Can you work these out from the model? Positions are in its coordinate system, mm. A direction names the side the tool comes from. Round coordinates to 2 decimals unless told otherwise and drop trailing zeros. Order: outer loops, then holes, each group sorted by start corner. A loop starts at its lowest first (then second) coordinate and runs counter-clockwise, first axis right, second up. Notation, with made-up numbers: (19, -8.75) - (34, -8.75) arc R21 ccw to (34, 5.25) - close; hole circle Ø6 at (-18.5, 32.25). An arc over 180 degrees is marked (long way). Write item = value, one per line.
from build123d import *

# Parameters (mm, degrees)
EXTRUDE_1_DEPTH        = 40
SKETCH_5_W             = 3
SKETCH_5_H             = 6
SKETCH_5_W_2           = 6
SKETCH_5_H_2           = 3
EXTRUDE_3_DEPTH        = 2.5
SKETCH_6_W             = 6
SKETCH_6_H             = 3
SKETCH_6_W_2           = 3
SKETCH_6_H_2           = 6
EXTRUDE_4_DEPTH        = 2.5
FILLET_1_R             = 1
CUT_EXTRUDE_8754_DEPTH = 7
CUT_EXTRUDE_START      = -7
CUT_EXTRUDE_9199_DEPTH = 7


with BuildPart() as part:
    # 草图2 → 凸台-拉伸1 (new body)
    with BuildSketch(Plane(origin=(0, 0, 0), x_dir=(1, 0, 0), z_dir=(0, 1, 0))):
        with BuildLine():
            Line((-33, 3.25), (-36.5, 3.25))
            Line((-36.5, 3.25), (-36.5, -3.25))
            Line((-36.5, -3.25), (-33, -3.25))
            ThreePointArc((-33, -3.25), (-34.3699608, -13.457697281), (-37.384420147, -23.305890579))
            ThreePointArc((-37.384420147, -23.305890579), (-35.741677738, -34.13030337), (-25.5, -38))
            Line((-25.5, -38), (-25.5, -41.5))
            Line((-25.5, -41.5), (-19, -41.5))
            Line((-19, -41.5), (-19, -38))
            ThreePointArc((-19, -38), (0, -34.737686486), (19, -38))
            Line((19, -38), (19, -41.5))
            Line((19, -41.5), (25.5, -41.5))
            Line((25.5, -41.5), (25.5, -38))
            ThreePointArc((25.5, -38), (35.741677738, -34.13030337), (37.384420147, -23.305890579))
            ThreePointArc((37.384420147, -23.305890579), (34.3699608, -13.457697281), (33, -3.25))
            Line((33, -3.25), (36.5, -3.25))
            Line((36.5, -3.25), (36.5, 3.25))
            Line((36.5, 3.25), (33, 3.25))
            ThreePointArc((33, 3.25), (34.3699608, 13.457697281), (37.384420147, 23.305890579))
            ThreePointArc((37.384420147, 23.305890579), (35.741677738, 34.13030337), (25.5, 38))
            Line((25.5, 38), (25.5, 41.5))
            Line((25.5, 41.5), (19, 41.5))
            Line((19, 41.5), (19, 38))
            ThreePointArc((19, 38), (0, 32.48661644), (-19, 38))
            Line((-19, 38), (-19, 41.5))
            Line((-19, 41.5), (-25.5, 41.5))
            Line((-25.5, 41.5), (-25.5, 38))
            ThreePointArc((-25.5, 38), (-35.741677738, 34.13030337), (-37.384420147, 23.305890579))
            ThreePointArc((-37.384420147, 23.305890579), (-34.3699608, 13.457697281), (-33, 3.25))
        make_face()
        with BuildLine():
            ThreePointArc((-24.584159113, 34.841334273), (-32.862117731, 33.087897358), (-34.944211337, 24.886432483))
            ThreePointArc((-34.944211337, 24.886432483), (-31.079757149, 0), (-34.944211337, -24.886432483))
            ThreePointArc((-34.944211337, -24.886432483), (-33.784066651, -32.031796166), (-27.335670062, -35.32122458))
            ThreePointArc((-27.335670062, -35.32122458), (0, -31.93514908), (27.335670062, -35.32122458))
            ThreePointArc((27.335670062, -35.32122458), (33.784066651, -32.031796166), (34.944211337, -24.886432483))
            ThreePointArc((34.944211337, -24.886432483), (31.079757149, 0), (34.944211337, 24.886432483))
            ThreePointArc((34.944211337, 24.886432483), (32.862117731, 33.087897358), (24.584159113, 34.841334273))
            ThreePointArc((24.584159113, 34.841334273), (0, 30.397281148), (-24.584159113, 34.841334273))
        make_face(mode=Mode.SUBTRACT)
    extrude(amount=-EXTRUDE_1_DEPTH)

    # 草图5 → 凸台-拉伸3 (add)
    with BuildSketch(Plane(origin=(0, 0, 0), x_dir=(1, 0, 0), z_dir=(0, 1, 0))):
        with Locations((-34.75, 0)):
            Rectangle(SKETCH_5_W, SKETCH_5_H)
        with Locations((-22.25, -39.75)):
            Rectangle(SKETCH_5_W_2, SKETCH_5_H_2)
        with Locations((-22.25, 39.75)):
            Rectangle(SKETCH_5_W_2, SKETCH_5_H_2)
        with Locations((22.25, 39.75)):
            Rectangle(SKETCH_5_W_2, SKETCH_5_H_2)
        with Locations((22.25, -39.75)):
            Rectangle(SKETCH_5_W_2, SKETCH_5_H_2)
        with Locations((34.75, 0)):
            Rectangle(SKETCH_5_W, SKETCH_5_H)
    extrude(amount=EXTRUDE_3_DEPTH)

    # 草图6 → 凸台-拉伸4 (add)
    with BuildSketch(Plane.XZ.offset(40)):
        with Locations((-22.25, 39.75)):
            Rectangle(SKETCH_6_W, SKETCH_6_H)
        with Locations((-34.75, 0)):
            Rectangle(SKETCH_6_W_2, SKETCH_6_H_2)
        with Locations((-22.25, -39.75)):
            Rectangle(SKETCH_6_W, SKETCH_6_H)
        with Locations((22.25, 39.75)):
            Rectangle(SKETCH_6_W, SKETCH_6_H)
        with Locations((22.25, -39.75)):
            Rectangle(SKETCH_6_W, SKETCH_6_H)
        with Locations((34.75, 0)):
            Rectangle(SKETCH_6_W_2, SKETCH_6_H_2)
    extrude(amount=EXTRUDE_4_DEPTH)

    # 圆角1
    fillet_1_edges = [part.edges().sort_by_distance(p)[0] for p in [
        (-25.5, -20, -38),
        (-19, -20, -38),
        (19, -20, -38),
        (25.5, -20, -38),
        (33, -20, -3.25),
        (33, -20, 3.25),
        (25.5, -20, 38),
        (19, -20, 38),
        (-19, -20, 38),
        (-25.5, -20, 38),
        (-33, -20, 3.25),
        (-33, -20, -3.25),
    ]]
    fillet(fillet_1_edges, radius=FILLET_1_R)

    # 草图7 → Cut-Extrude 8754 (cut)
    with BuildSketch(Plane(origin=(0, 0, 0), x_dir=(1, 0, 0), z_dir=(0, 1, 0))):
        with BuildLine():
            Line((-36.633725749, -21.323718343), (-33.898557891, -21.323718343))
            ThreePointArc((-33.898557891, -21.323718343), (-34.401232724, -23.110989975), (-34.944211337, -24.886432483))
            ThreePointArc((-34.944211337, -24.886432483), (-35.274550553, -28.150449442), (-34.273344825, -31.274632183))
            Line((-34.273344825, -31.274632183), (-37.421883074, -31.274632183))
            ThreePointArc((-37.421883074, -31.274632183), (-38.165581654, -27.580951917), (-37.605977079, -23.854934713))
            ThreePointArc((-37.605977079, -23.854934713), (-37.106234952, -22.594556671), (-36.633725749, -21.323718343))
        make_face()
        with BuildLine():
            Line((36.633725749, -21.323718343), (33.898557891, -21.323718343))
            ThreePointArc((33.898557891, -21.323718343), (34.401232724, -23.110989975), (34.944211337, -24.886432483))
            ThreePointArc((34.944211337, -24.886432483), (35.274550553, -28.150449442), (34.273344825, -31.274632183))
            Line((34.273344825, -31.274632183), (37.421883074, -31.274632183))
            ThreePointArc((37.421883074, -31.274632183), (38.165581654, -27.580951917), (37.605977079, -23.854934713))
            ThreePointArc((37.605977079, -23.854934713), (37.106234952, -22.594556671), (36.633725749, -21.323718343))
        make_face()
        with BuildLine():
            Line((-36.633725749, 21.323718343), (-33.898557891, 21.323718343))
            ThreePointArc((-33.898557891, 21.323718343), (-34.401232724, 23.110989975), (-34.944211337, 24.886432483))
            ThreePointArc((-34.944211337, 24.886432483), (-35.274550553, 28.150449442), (-34.273344825, 31.274632183))
            Line((-34.273344825, 31.274632183), (-37.421883074, 31.274632183))
            ThreePointArc((-37.421883074, 31.274632183), (-38.165581654, 27.580951917), (-37.605977079, 23.854934713))
            ThreePointArc((-37.605977079, 23.854934713), (-37.106234952, 22.594556671), (-36.633725749, 21.323718343))
        make_face()
        with BuildLine():
            Line((37.421883074, 31.274632183), (34.273344825, 31.274632183))
            ThreePointArc((34.273344825, 31.274632183), (35.274550553, 28.150449442), (34.944211337, 24.886432483))
            ThreePointArc((34.944211337, 24.886432483), (34.401232724, 23.110989975), (33.898557891, 21.323718343))
            Line((33.898557891, 21.323718343), (36.633725749, 21.323718343))
            ThreePointArc((36.633725749, 21.323718343), (37.106234952, 22.594556671), (37.605977079, 23.854934713))
            ThreePointArc((37.605977079, 23.854934713), (38.165581654, 27.580951917), (37.421883074, 31.274632183))
        make_face()
    extrude(amount=-CUT_EXTRUDE_8754_DEPTH, mode=Mode.SUBTRACT)

    # 草图8 → Cut-Extrude 9199 (cut)
    with BuildSketch(Plane.XZ.offset(40).offset(CUT_EXTRUDE_START)):
        with BuildLine():
            Line((-33.167247328, -5.619996041), (-31.272419616, -5.619996041))
            ThreePointArc((-31.272419616, -5.619996041), (-31.726152882, -10.279804399), (-32.444885624, -14.906154046))
            Line((-32.444885624, -14.906154046), (-34.704557814, -14.906154046))
            ThreePointArc((-34.704557814, -14.906154046), (-33.762273508, -10.291819093), (-33.167247328, -5.619996041))
        make_face()
        with BuildLine():
            Line((-34.704557814, 14.906154046), (-32.444885624, 14.906154046))
            ThreePointArc((-32.444885624, 14.906154046), (-31.726152882, 10.279804399), (-31.272419616, 5.619996041))
            Line((-31.272419616, 5.619996041), (-33.167247328, 5.619996041))
            ThreePointArc((-33.167247328, 5.619996041), (-33.762273508, 10.291819093), (-34.704557814, 14.906154046))
        make_face()
        with BuildLine():
            Line((33.167247328, -5.619996041), (31.272419616, -5.619996041))
            ThreePointArc((31.272419616, -5.619996041), (31.726152882, -10.279804399), (32.444885624, -14.906154046))
            Line((32.444885624, -14.906154046), (34.704557814, -14.906154046))
            ThreePointArc((34.704557814, -14.906154046), (33.762273508, -10.291819093), (33.167247328, -5.619996041))
        make_face()
        with BuildLine():
            Line((33.167247328, 5.619996041), (31.272419616, 5.619996041))
            ThreePointArc((31.272419616, 5.619996041), (31.726152882, 10.279804399), (32.444885624, 14.906154046))
            Line((32.444885624, 14.906154046), (34.704557814, 14.906154046))
            ThreePointArc((34.704557814, 14.906154046), (33.762273508, 10.291819093), (33.167247328, 5.619996041))
        make_face()
    extrude(amount=CUT_EXTRUDE_9199_DEPTH, mode=Mode.SUBTRACT)


solid = part.part
(1) If I drill on line 1 (X direction, y = -6, z = -0.5); line 2 (Y direction, x = -15, z = 35); line 3 (Z direction, x = 7, y = -34.5), over which ranges is the centre line in solid material (lowest first)? Write a range as from..to.
Computed:
line_1 = -36.5..-31.08, 31.08..36.5
line_2 = -40..0
line_3 = -33.18..-30.75, 32.15..35.17
(2) If we section it at D-D (x = -2): Write out the boundary of the cut face in (y, z).
Computed:
outline = (-40, -32.54) - (0, -32.54) - (0, -30.43) - (-40, -30.43) - close; (-40, 31.95) - (0, 31.95) - (0, 34.77) - (-40, 34.77) - close
(3) If we section it at C-C (z = -26.5): Write out the boundary of the cut face in (x, y), plus the area to 3 significant figures.
Computed:
outline = (-38.12, -40) - (-35.28, -40) - (-35.28, -7) - (-38.12, -7) - close; (35.28, -40) - (38.12, -40) - (38.12, -7) - (35.28, -7) - close
area = 188 mm^2
(4) On a 3-axis mill with a long thin cutter (end or side, diameter ignored), from which of +Z, -Z, +X, -X, +Y, -Y can I reach the whole of each face in a straight line? I mean faces 5 (the face through (-35, -20, 3.25)), 6 (the face through (34, -36, -14.906)), 7 (the face through (35, -3, -21.324)). Say none if no direction works.
Computed:
face_5 = -X, +Y, -Y
face_6 = +X, -X, -Y
face_7 = +X, -X, +Y
(5) If we section it at A-A (x = -22): Write out the boundary of the cut face in (y, z).
Computed:
outline = (-42.5, -41.25) - (-40, -41.25) - (-40, -41.5) - (0, -41.5) - (0, -41.25) - (2.5, -41.25) - (2.5, -38.25) - (0, -38.25) - (0, -33.93) - (-40, -33.93) - (-40, -38.25) - (-42.5, -38.25) - close; (-42.5, 38.25) - (-40, 38.25) - (-40, 34.12) - (0, 34.12) - (0, 38.25) - (2.5, 38.25) - (2.5, 41.25) - (0, 41.25) - (0, 41.5) - (-40, 41.5) - (-40, 41.25) - (-42.5, 41.25) - close
(6) Thinking about a two-plate mould opening in Z: for faces 1 (the face through (-35, -3, 21.324)), 2 (the face through (-25.25, -41, 40)), 3 (the face through (-0.26, -19.72, 34.74)), 4 (the face through (-22, -41, 38.25)), which applies, +Z half, -Z half, draft (parallel to the pull), parting line (faces both ways), or undercut?
Computed:
face_1 = undercut
face_2 = draft
face_3 = +Z half
face_4 = undercut
(7) Will these pins go through, and if not, where does the flat tip stop? P1, Ø8, axis at x = 3.5, y = -30.5, coming from the +Z side; P2, Ø0.8, axis at x = 21.5, y = -41.5, coming from the +Z side; P3, Ø3, axis at x = 29, y = -26.5, coming from the -Z side; P4, Ø10, axis at x = 18, y = -9, coming from the -Z side.
Computed:
P1 = 35.23
P2 = 41.25
P3 = -38.15
P4 = -41.5
(8) If we section it at B-B (z = -2): Write out the boundary of the cut face in (x, y).
Computed:
outline = (-36.5, -40) - (-36.25, -40) - (-36.25, -42.5) - (-33.25, -42.5) - (-33.25, -40) - (-31.1, -40) - (-31.1, 0) - (-33.25, 0) - (-33.25, 2.5) - (-36.25, 2.5) - (-36.25, 0) - (-36.5, 0) - close; (31.1, -40) - (33.25, -40) - (33.25, -42.5) - (36.25, -42.5) - (36.25, -40) - (36.5, -40) - (36.5, 0) - (36.25, 0) - (36.25, 2.5) - (33.25, 2.5) - (33.25, 0) - (31.1, 0) - close
